Geometry check sheet. Reference: drawing and pictorial views, mm from the part's lowest x, y, z. A direction names the side the tool comes from. Round coordinates to 2 decimals unless told otherwise and drop trailing zeros. Order: outer loops, then holes, each group sorted by start corner. A loop starts at its lowest first (then second) coordinate and runs counter-clockwise, first axis right, second up.
Q1. Depth check by flat-ended pin: P1, Ø2, axis at x = 72, z = 28, coming from the -Y side; P2, Ø12, axis at x = 11.5, z = 20.5, coming from the -Y side; P3, Ø13.5, axis at x = 78.5, z = 20.5, coming from the -Y side; P4, Ø5, axis at y = 13, z = 6.5, coming from the -X side. Enter the tip coordinate at first touch or a pass-through.
Q2. Scan lines: probe 1 along X at (y, z) = (19, 10) (1 decimal); probe 2 along X at (y, z) = (22.5, 6) (1 decimal). Record each from-to range of solid material in increasing order.
Q3. Mould release check, pull along Z, two halves, no side actions. Record for the marked faces 1, 2 and 3: +Z half, -Z half, draft (parallel to the pull), parting line (faces both ways), or undercut.
Q4. Cross-section at B-B on y = 22. Record the cut outline in (x, z).
Q5. Set-up check for the marked faces 4, 5 and 6: record each of +Z, -Z, +X, -X, +Y, -Y from which the full face is reachable in a straight line by a thin tool's end or side.
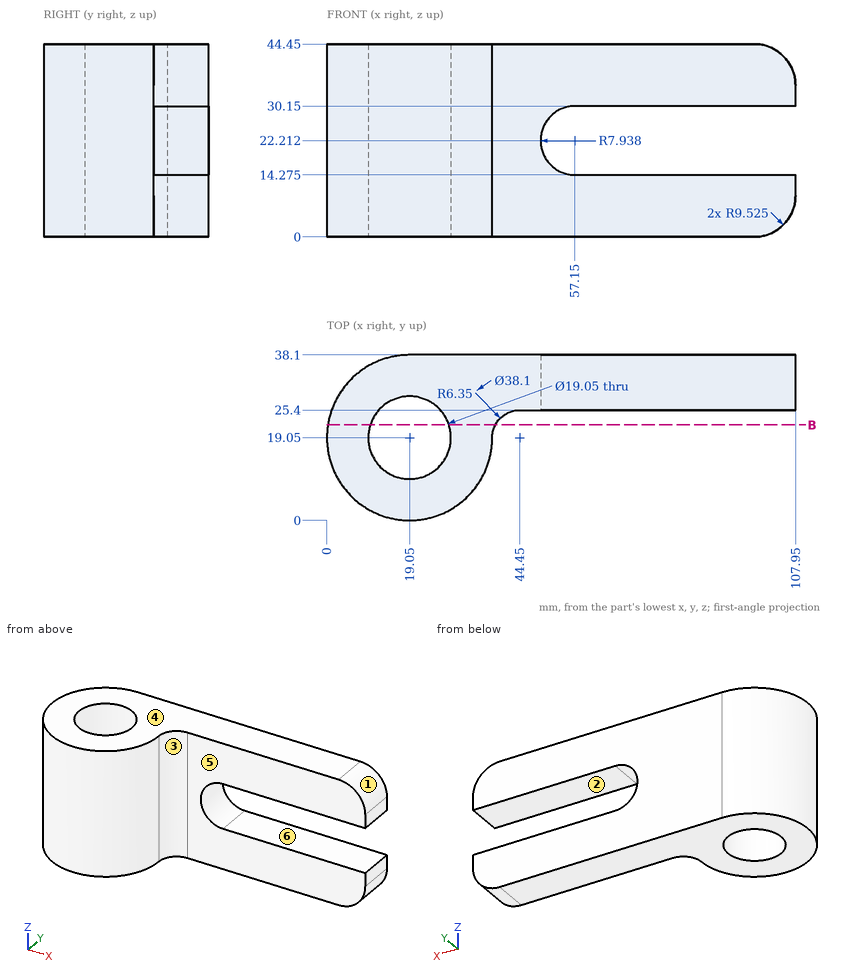
Results found:
1. P1: passes through
1. P2: stops at y = 0.06
1. P3: stops at y = 25.4
1. P4: stops at x = 0.33
2. probe 1: x = 0 to 9.5, 28.6 to 38.1
2. probe 2: x = 0.3 to 10.2, 27.9 to 39.1
3. face 1: +Z half
3. face 2: undercut
3. face 3: draft
4. outline: (0.23, 0) - (9.99, 0) - (9.99, 44.45) - (0.23, 44.45) - close; (28.11, 0) - (38.83, 0) - (38.83, 44.45) - (28.11, 44.45) - close
5. face 4: +Z, +X, -X, +Y, -Y
5. face 5: +Z, -Z, +X, -Y
5. face 6: +X, +Y, -Y
